from build123d import *

# Parameters (mm, degrees)
F0_W     = 180.34
F0_H     = 174.487158
F1_DEPTH = 6.35
F2_R     = 5.08
F3_W     = 95.25
F3_H     = 152.4
F4_DEPTH = 0.254
F3_R     = 6.35
F5_DEPTH = 25.4


with BuildPart() as f1:
    # F0 (on Top) → F1 (new body)
    with BuildSketch(Plane.XY):
        with Locations((-7.8691, -48.399139)):
            Rectangle(F0_W, F0_H)
    extrude(amount=F1_DEPTH)

    # F2
    f2_edges = [f1.edges().sort_by_distance(p)[0] for p in [
        (-98.0391, -135.642718, 3.175),
        (82.3009, -135.642718, 3.175),
        (-98.0391, 38.84444, 3.175),
        (82.3009, 38.84444, 3.175),
    ]]
    fillet(f2_edges, radius=F2_R)

    # F3 (on face) → F4 (cut)
    with BuildSketch(Plane.XY.offset(6.35)):
        with Locations((-40.792745, -48.399139)):
            Rectangle(F3_W, F3_H)
    extrude(amount=-F4_DEPTH, mode=Mode.SUBTRACT)

    # F3 (on face) → F5 (cut)
    with BuildSketch(Plane.XY.offset(6.35)):
        with Locations((37.122272, -121.842124)):
            Circle(F3_R)
        with Locations((37.122272, -73.836124)):
            Circle(F3_R)
        with Locations((37.122272, 22.175876)):
            Circle(F3_R)
        with Locations((37.122272, -25.830124)):
            Circle(F3_R)
    extrude(amount=-F5_DEPTH, mode=Mode.SUBTRACT)


solid = f1.part
The model under review builds one solid part; all positions refer to its coordinate system, in mm. A direction names the side the tool comes from. Round coordinates to 2 decimals unless told otherwise and drop trailing zeros. Loops run counter-clockwise (first coordinate to the right, second up) from the corner with the lowest first, then second, coordinate; pieces in that order, holes last. Notation, with made-up numbers: (88.25, -34) -> (142.25, -34) arc R6 cw to (142.25, -24) -> close; hole circle Ø6 at (56, 52). An arc over 180 degrees is marked (long way). Return JSON: item names as keys, results as strings.
(1) Add section B-B on z = 2. Write out the cut boundary in (x, y).
Solved:
{"outline": "(-98.04, -130.56) arc R5.08 ccw to (-92.96, -135.64) -> (77.22, -135.64) arc R5.08 ccw to (82.3, -130.56) -> (82.3, 33.76) arc R5.08 ccw to (77.22, 38.84) -> (-92.96, 38.84) arc R5.08 ccw to (-98.04, 33.76) -> close; hole circle Ø12.7 at (37.12, -121.84); hole circle Ø12.7 at (37.12, -73.84); hole circle Ø12.7 at (37.12, -25.83); hole circle Ø12.7 at (37.12, 22.18)"}
(2) For pin 1 (10 mm diameter, centred on x = -6, y = -6, fed in from +Z), flat-tipped, find the tip position at first contact; note if it passes through.
Solved:
{"pin 1": "z = 6.1"}
(3) For line 1 (X direction, y = -124.5, z = 3.5); line 2 (X direction, y = -127, z = 3.75); line 3 (Z direction, x = 2, y = -102), list the stretches that pass through material, from the lowest coordinate up.
Solved:
{"line 1": "-98.04 to 31.36, 42.89 to 82.3", "line 2": "-98.04 to 33.42, 40.83 to 82.3", "line 3": "0 to 6.1"}
(4) Add section C-C on y = -98. Write out the cut boundary in (x, z).
Solved:
{"outline": "(-98.04, 0) -> (82.3, 0) -> (82.3, 6.35) -> (6.83, 6.35) -> (6.83, 6.1) -> (-88.42, 6.1) -> (-88.42, 6.35) -> (-98.04, 6.35) -> close"}
(5) For faces 1 (the flat face through (-41, -47, 6.096)), 2 (the cylindrical face through (80.85, 37.32, 3.22)), list the 3-axis set-ups (+Z, -Z, +X, -X, +Y, -Y) from which the entire face can be reached by the end or side of a thin tool; tool diameter is ignored.
Solved:
{"face 1": "+Z", "face 2": "+Z, -Z, +X, +Y"}
(6) The part is to be moulded in two halves that separate along Y. For faces 3 (the cylindrical face through (35.746, -80.035, 3.219)), 4 (the cylindrical face through (35.746, 15.977, 3.219)), 5 (the flat face through (-9, -135.643, 3)), 6 (the cylindrical face through (-96.59, 37.32, 3.22)), say which applies: released by +Y, released by -Y, zero draft, split by the parting line, or undercut.
Solved:
{"face 3": "undercut", "face 4": "undercut", "face 5": "released by -Y", "face 6": "released by +Y"}
(7) Add section A-A on x = -56. Write out the cut boundary in (y, z).
Solved:
{"outline": "(-135.64, 0) -> (38.84, 0) -> (38.84, 6.35) -> (27.8, 6.35) -> (27.8, 6.1) -> (-124.6, 6.1) -> (-124.6, 6.35) -> (-135.64, 6.35) -> close"}
